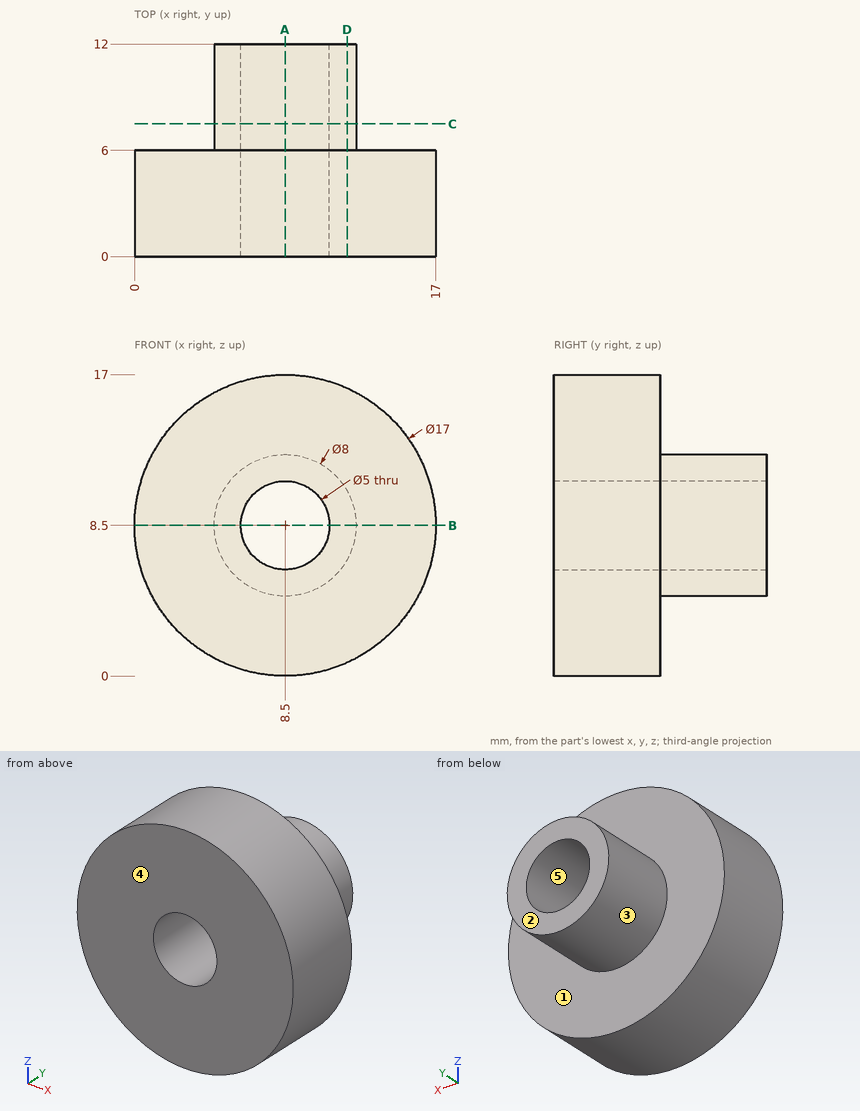
Part print with two shaded views. Sizes in mm from the minimum x, y, z corner. A direction names the side the tool comes from. Coordinates: 2 decimals unless noted, no trailing zeros. Write each loop counter-clockwise with the first axis right and the second up, starting at its lowest first coordinate (ties: lowest second). Pieces come first, ordered by that corner, then holes. Notation, with made-up numbers: (56.5, 3.25) - (73.5, 3.25) arc R31 ccw to (73.5, 37.25) - close; hole circle Ø10 at (73.25, -39). An arc over 180 degrees is marked (long way). Put each result on its own line as item: value.
1. 3-axis set-ups, long thin cutter, end or side, ignore diameter. For the marked faces 1 and 2: which of +Z, -Z, +X, -X, +Y, -Y reach the whole face in a straight line?
Final values:
face 1: +Y
face 2: +Z, -Z, +X, -X, +Y
2. Flat gauge pins, fed straight in: pin 1 Ø2 at (x, z) = (6, 6) entering from -Y; pin 2 Ø4 at (x, y) = (4.5, 5.5) entering from +Z; pin 3 Ø1.5 at (x, y) = (6.5, 3) entering from -Z. Where does each tip first touch, or does it go through?
Final values:
pin 1: stops at y = 0
pin 2: stops at z = 16.76
pin 3: stops at z = 0.09
3. Band-saw the part on C-C (y = 7.5). Write the cut outline in (x, z), then the cut area to 3 significant figures.
Final values:
outline: circle Ø8 at (8.5, 8.5); hole circle Ø5 at (8.5, 8.5)
area: 30.6 mm²
4. Band-saw the part on B-B (z = 8.5). Write the cut outline in (x, y).
Final values:
outline: (0, 0) - (6, 0) - (6, 12) - (4.5, 12) - (4.5, 6) - (0, 6) - close; (11, 0) - (17, 0) - (17, 6) - (12.5, 6) - (12.5, 12) - (11, 12) - close
5. Band-saw the part on A-A (x = 8.5). Write the cut outline in (y, z), then the cut area to 3 significant figures.
Final values:
outline: (0, 0) - (6, 0) - (6, 4.5) - (12, 4.5) - (12, 6) - (0, 6) - close; (0, 11) - (12, 11) - (12, 12.5) - (6, 12.5) - (6, 17) - (0, 17) - close
area: 90.0 mm²
6. Two-plate mould, pull along Z, no slides. Class the marked faces 3, 4 and 5: +Z half, -Z half, draft (parallel to the pull), parting line (faces both ways), or undercut.
Final values:
face 3: parting line
face 4: draft
face 5: undercut
7. Probe line 1 along X through (y, z) = (5, 8.5); line 2 along X through (y, z) = (9, 8.5); line 3 along Y through (x, z) = (13.5, 5.25). List the from-to ranges inside material, lowest first. Write a range as [from, to].
Final values:
line 1: x = [0, 6], [11, 17]
line 2: x = [4.5, 6], [11, 12.5]
line 3: y = [0, 6]
8. Band-saw the part on D-D (x = 12). Write the cut outline in (y, z).
Final values:
outline: (0, 0.75) - (6, 0.75) - (6, 6.56) - (12, 6.56) - (12, 10.44) - (6, 10.44) - (6, 16.25) - (0, 16.25) - close
